Verification items for this drawing (mm, ordinates from the low corner). Round coordinates to 2 decimals unless told otherwise and drop trailing zeros. Loops run counter-clockwise (first coordinate to the right, second up) from the corner with the lowest first, then second, coordinate; pieces in that order, holes last. Notation, with made-up numbers: M 46,61.5 L 91,61.5 A17 ccw 91,85.5 Z; hole C 42.5,-12 d1. An arc over 180 degrees is marked long. One line per item, written item: value.
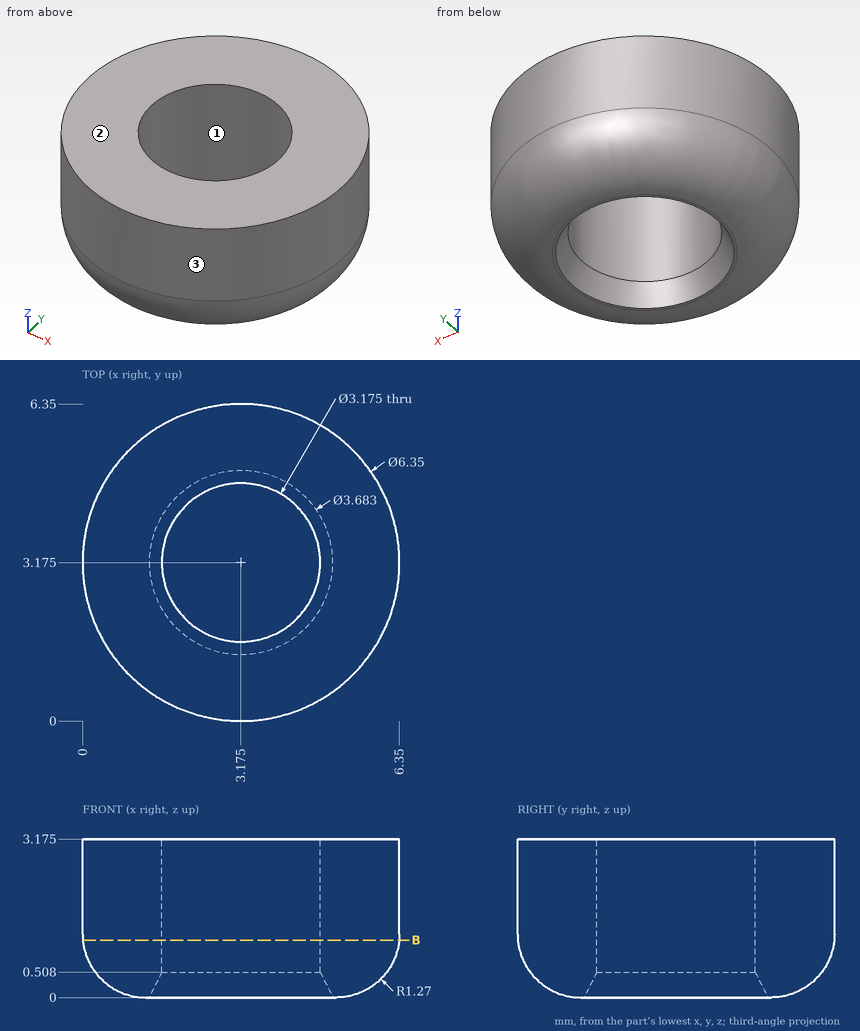
(1) Thickness scan on L1, parallel to Z at x = 2.75, y = 1.25 (3 decimals); L2, parallel to X at y = 3, z = 0.4; L3, parallel to Y at x = 1.75, z = 2.75. Record the ranges inside material, lowest first. Write a range as from..to.
Completed:
L1: z = 0.002..3.175
L2: x = 0.35..1.54, 4.81..6
L3: y = 0.34..2.48, 3.87..6.01
(2) Depth check by flat-ended pin: pin 1 Ø1 at (y, z) = (5.5, 2.5) entering from -X; pin 2 Ø1.5 at (y, z) = (4.5, 2.5) entering from +X; pin 3 Ø3.5 at (x, y) = (3.175, 3.175) entering from +Z (3 decimals). Enter the tip coordinate at first touch or a pass-through.
Completed:
pin 1: stops at x = 0.58
pin 2: stops at x = 6.3
pin 3: stops at z = 3.175
(3) Mould release check, pull along X, two halves, no side actions. Record for the marked faces 1, 2 and 3: +X half, -X half, draft (parallel to the pull), parting line (faces both ways), or undercut.
Completed:
face 1: undercut
face 2: draft
face 3: parting line
(4) Sectioned sample at B-B on z = 1.15. Enter the section's corners in (x, y) (1 decimal).
Completed:
outline: C 3.2,3.2 d6.3; hole C 3.2,3.2 d3.2
